Geometry: see drawing. Coordinates: mm, zero at the bounding-box minimum. Coordinates: 2 decimals unless noted, no trailing zeros. Write each loop counter-clockwise with the first axis right and the second up, starting at its lowest first coordinate (ties: lowest second). Pieces come first, ordered by that corner, then holes. Notation, with made-up numbers: M 61.5,73 L 98.5,73 A17 ccw 98.5,80 Z; hole C 38,86.5 d2. An arc over 180 degrees is marked long. One line per item, written item: value. Start each with the question number.
Item 1: Cut plane B-B, the plane z = 3.75. Output: boundary loops of the cut face in (x, y), then the cut area to 3 significant figures.
Item 2: Cut plane A-A, the plane y = 0.6. Output: boundary loops of the cut face in (x, z).
Item 3: Ray query, L1, parallel to Z at x = 1.5, y = 2; L2, parallel to X at y = 9.25, z = 1.25. Return the intervals inside material, ascending. Write a range as from..to.
Item 4: Cut plane C-C, the plane x = 19.4. Output: boundary loops of the cut face in (y, z).
Item 5: Cut plane D-D, the plane y = 7.5. Output: boundary loops of the cut face in (x, z), then the cut area to 3 significant figures.
Item 6: Pin query (flat end, axial travel): P1, Ø1.5, axis at y = 4.5, z = 6, coming from the -X side; P2, Ø2, axis at x = 14, y = 6, coming from the -Z side. Return the tip coordinate at first contact, or that it passes through.
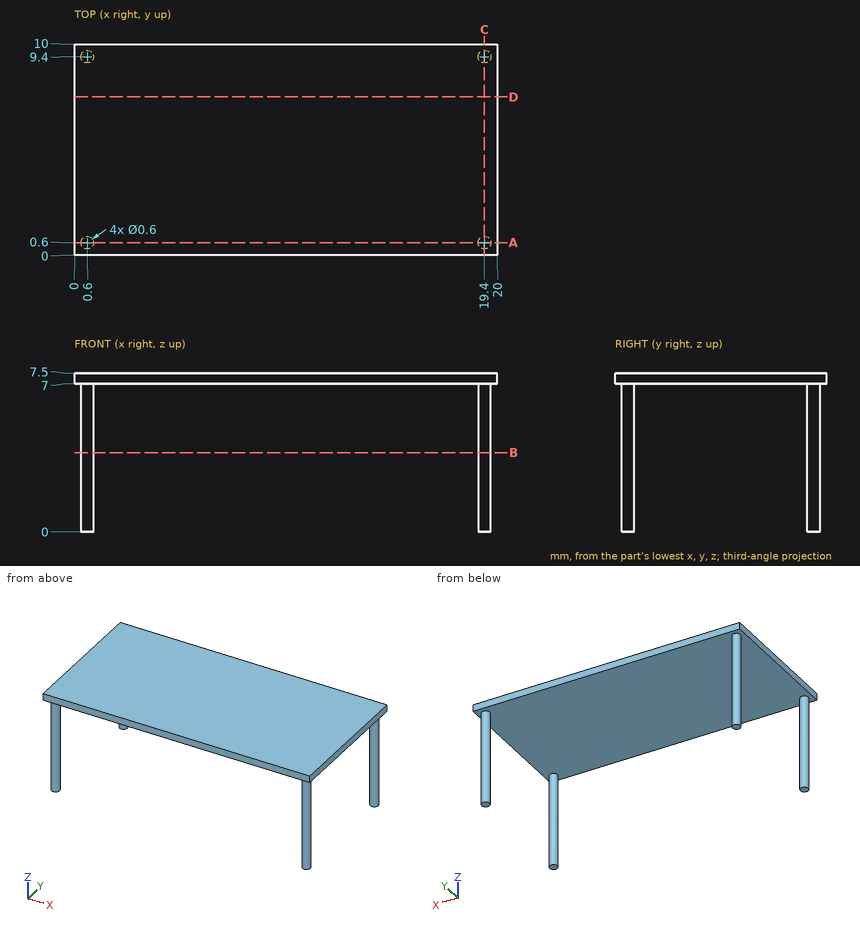
From the geometry:
1. outline: C 0.6,0.6 d0.6; C 0.6,9.4 d0.6; C 19.4,0.6 d0.6; C 19.4,9.4 d0.6
1. area: 1.13 mm²
2. outline: M 0,7 L 0.3,7 L 0.3,0 L 0.9,0 L 0.9,7 L 19.1,7 L 19.1,0 L 19.7,0 L 19.7,7 L 20,7 L 20,7.5 L 0,7.5 Z
3. L1: z = 7..7.5
3. L2: x = 0.34..0.86, 19.14..19.66
4. outline: M 0,7 L 0.3,7 L 0.3,0 L 0.9,0 L 0.9,7 L 9.1,7 L 9.1,0 L 9.7,0 L 9.7,7 L 10,7 L 10,7.5 L 0,7.5 Z
5. outline: M 0,7 L 20,7 L 20,7.5 L 0,7.5 Z
5. area: 10.0 mm²
6. P1: passes through
6. P2: stops at z = 7
